Work out the finished part from the listing and answer in its coordinate system (mm). Face numbers are marked on the shaded views. Round coordinates to 2 decimals unless told otherwise and drop trailing zeros. Write each loop counter-clockwise with the first axis right and the second up, starting at its lowest first coordinate (ties: lowest second). Pieces come first, ordered by that corner, then holes. Notation, with made-up numbers: (2, -32.75) - (29, -32.75) arc R28 cw to (29, -12.75) - close; hole circle Ø1 at (28.5, -30.5). An arc over 180 degrees is marked (long way). Write item = value, one per line. Start each with the question number.
from build123d import *

# Parameters (mm, degrees)
CROQUIS1_W              = 60
CROQUIS1_H              = 20
SALIENTE_EXTRUIR1_DEPTH = 20
VACIADO1_T              = 1.5
CORTAR_EXTRUIR1_DEPTH   = 18
CROQUIS3_R              = 1.25
CORTAR_EXTRUIR2_DEPTH   = 2.5


with BuildPart() as part:
    # Croquis1 → Saliente-Extruir1 (new body)
    with BuildSketch(Plane(origin=(0, 0, 0), x_dir=(1, 0, 0), z_dir=(0, 1, 0))):
        with Locations((30, -10)):
            Rectangle(CROQUIS1_W, CROQUIS1_H)
    extrude(amount=SALIENTE_EXTRUIR1_DEPTH)

    # Vaciado1 (no face opened: a closed hollow body)
    add(offset(amount=-VACIADO1_T, mode=Mode.PRIVATE), mode=Mode.SUBTRACT)

    # Croquis2 → Cortar-Extruir1 (cut)
    with BuildSketch(Plane(origin=(0, 20, 0), x_dir=(1, 0, 0), z_dir=(0, 1, 0))):
        Polygon((1.5, -2.5), (21.5, -2.5), (21.5, -8.5), (56.5, -8.5), (56.5, -11.5), (21.5, -11.5), (21.5, -17.5), (1.5, -17.5), align=None)
    extrude(amount=-CORTAR_EXTRUIR1_DEPTH, mode=Mode.SUBTRACT)

    # Croquis3 → Cortar-Extruir2 (cut, through all)
    with BuildSketch(Plane(origin=(0, 1.5, 0), x_dir=(1, 0, 0), z_dir=(0, 1, 0))):
        with Locations(Location((4, -10.25, 0), (0, 0, 270))):  # turned: the seam where the file's is
            Circle(CROQUIS3_R)
    extrude(amount=-CORTAR_EXTRUIR2_DEPTH, mode=Mode.SUBTRACT)


solid = part.part
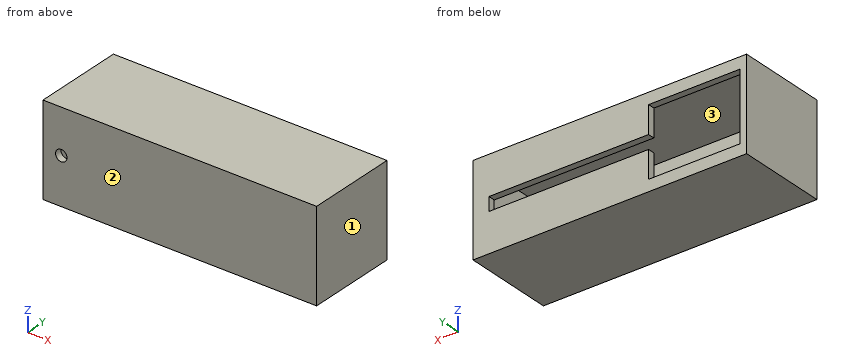
1. Find section B-B on z = 10.25. Give the vertices of the cut face in (x, y), plus the area to 3 significant figures.
2. Find section C-C on y = 6.25. Give the vertices of the cut face in (x, z), plus the area to 3 significant figures.
3. Consider line 1 (Z direction, x = 36.5, y = 16.75); line 2 (X direction, y = 7, z = 1.75). Determine where each line is inside the solid, lowest interval first.
4. Find section A-A on x = 4. Give the vertices of the cut face in (y, z).
5. Find section D-D on x = 27. Give the vertices of the cut face in (y, z).
6. For a pull along Y with two mould halves and no side action, classify the marked faces 1, 2 and 3 as released by +Y, released by -Y, zero draft, split by the parting line, or undercut.
Answer key:
q1.outline = (0, 0) - (2.75, 0) - (2.75, 1.5) - (1.5, 1.5) - (1.5, 20) - (0, 20) - close; (5.25, 0) - (60, 0) - (60, 20) - (56.5, 20) - (56.5, 18.5) - (58.5, 18.5) - (58.5, 1.5) - (5.25, 1.5) - close
q1.area = 145 mm²
q2.outline = (0, 0) - (60, 0) - (60, 20) - (0, 20) - close; hole (1.5, 1.5) - (58.5, 1.5) - (58.5, 18.5) - (1.5, 18.5) - close
q2.area = 231 mm²
q3.line_1 = 0 to 1.5, 18.5 to 20
q3.line_2 = 0 to 1.5, 58.5 to 60
q4.outline = (0, 0) - (20, 0) - (20, 2.5) - (18.5, 2.5) - (18.5, 1.5) - (1.5, 1.5) - (1.5, 9) - (0, 9) - close; (0, 11.5) - (1.5, 11.5) - (1.5, 18.5) - (18.5, 18.5) - (18.5, 17.5) - (20, 17.5) - (20, 20) - (0, 20) - close
q5.outline = (0, 0) - (20, 0) - (20, 8.5) - (18.5, 8.5) - (18.5, 1.5) - (1.5, 1.5) - (1.5, 18.5) - (18.5, 18.5) - (18.5, 11.5) - (20, 11.5) - (20, 20) - (0, 20) - close
q6.face_1 = zero draft
q6.face_2 = released by -Y
q6.face_3 = undercut
